Verification items for the finished model (mm, model axes). Face numbers are marked on the shaded views. A direction names the side the tool comes from. Coordinates: 2 decimals unless noted, no trailing zeros. Order: outer loops, then holes, each group sorted by start corner. A loop starts at its lowest first (then second) coordinate and runs counter-clockwise, first axis right, second up.
Q1. Draft check along Z on the marked faces 4, 5, 6 and 7. Enter one of: pulls with the +Z half, pulls with the -Z half, needs draft (parallel to the pull), parting line crosses it, or undercut.
Q2. Depth check by flat-ended pin: P1, Ø0.8, axis at x = 8, z = 20, coming from the -Y side; P2, Ø0.7, axis at x = -0.5, z = 12, coming from the +Y side; P3, Ø2.5, axis at y = 73.19, z = 6.34, coming from the -X side; P4, Ø3.5, axis at x = 0, z = 12, coming from the +Y side. Enter the tip coordinate at first touch or a pass-through.
Q3. Thickness scan on line 1 (X direction, y = 2, z = 20); line 2 (Z direction, x = 0, y = 7.75); line 3 (X direction, y = 34.5, z = 23). Record the ranges inside material, lowest first.
Q4. Cross-section at D-D, the plane z = 35. Record the boundary of the cut face in (x, y), and give its area (3 significant figures).
Q5. Cross-section at A-A, the plane x = -3. Record the boundary of the cut face in (y, z), and give its area (3 significant figures).
Q6. Cross-section at B-B, the plane x = 24. Count the separate pieces of the cut face and the enclosed holes in it, and give its area (3 significant figures).
Q7. Set-up check for the marked faces 1, 2 and 3: record each of +Z, -Z, +X, -X, +Y, -Y from which the full face is reachable in a straight line by a thin tool's end or side.
from build123d import *

# Parameters (mm, degrees)
DODANIE_WYCI_GNI_CIE1_DEPTH = 40
SZKIC2_R                    = 4.25
WYTNIJ_WYCI_GNI_CIE1_DEPTH  = 59
SZKIC3_R                    = 4.25
SZKIC3_R_2                  = 0.65
WYTNIJ_WYCI_GNI_CIE2_DEPTH  = 11
SZKIC4_R                    = 0.75
WYTNIJ_WYCI_GNI_CIE3_DEPTH  = 59
SZKIC3_3_R                  = 1.15
WYTNIJ_WYCI_GNI_CIE4_DEPTH  = 4


with BuildPart() as part:
    # Szkic1 → Dodanie-wyci_gni_cie1 (new body)
    with BuildSketch(Plane.XY):
        Polygon((21, 10), (-21, 10), (-21, 80), (-29, 80), (-29, 0), (29, 0), (29, 80), (21, 80), align=None)
    extrude(amount=DODANIE_WYCI_GNI_CIE1_DEPTH)

    # Szkic2 → Wytnij-wyci_gni_cie1 (cut, through all)
    with BuildSketch(Plane(origin=(29, 0, 0), x_dir=(0, 0, -1), z_dir=(1, 0, 0))):
        with BuildLine():
            ThreePointArc((-23.582337322, 70.675180947), (-10.416972499, 79.431921725), (0, 67.536795667))
            Line((0, 67.536795667), (0, 80))
            Line((0, 80), (-40, 80))
            Line((-40, 80), (-40, 14.688889066))
            ThreePointArc((-40, 14.688889066), (-38.089938994, 25.648227934), (-32.584991767, 35.315233546))
            ThreePointArc((-32.584991767, 35.315233546), (-26.211441646, 46.507556061), (-24, 59.196123761))
            Line((-24, 59.196123761), (-24, 67.536795667))
            ThreePointArc((-24, 67.536795667), (-23.895126058, 69.119823168), (-23.582337322, 70.675180947))
        make_face()
        with Locations((-12, 67.536795667)):
            Circle(SZKIC2_R)
    extrude(amount=-WYTNIJ_WYCI_GNI_CIE1_DEPTH, mode=Mode.SUBTRACT)

    # Szkic3 → Wytnij-wyci_gni_cie2 (cut, through all)
    with BuildSketch(Plane(origin=(0, 10, 0), x_dir=(1, 0, 0), z_dir=(0, 1, 0))):
        with Locations((0, -20)):
            Circle(SZKIC3_R)
        with Locations((5.656854249, -25.656854249)):
            Circle(SZKIC3_R_2)
        with Locations((8, -20)):
            Circle(SZKIC3_R_2)
        with Locations((0, -28)):
            Circle(SZKIC3_R_2)
        with Locations((-5.656854249, -25.656854249)):
            Circle(SZKIC3_R_2)
        with Locations((-8, -20)):
            Circle(SZKIC3_R_2)
        with Locations((-5.656854249, -14.343145751)):
            Circle(SZKIC3_R_2)
        with Locations((0, -12)):
            Circle(SZKIC3_R_2)
        with Locations((5.656854249, -14.343145751)):
            Circle(SZKIC3_R_2)
    extrude(amount=-WYTNIJ_WYCI_GNI_CIE2_DEPTH, mode=Mode.SUBTRACT)

    # Szkic4 → Wytnij-wyci_gni_cie3 (cut, through all)
    with BuildSketch(Plane.ZY.offset(29)):
        with Locations((12, 59.536795667)):
            Circle(SZKIC4_R)
        with Locations((6.343145751, 61.879941418)):
            Circle(SZKIC4_R)
        with Locations((4, 67.536795667)):
            Circle(SZKIC4_R)
        with Locations((6.343145751, 73.193649917)):
            Circle(SZKIC4_R)
        with Locations((12, 75.536795667)):
            Circle(SZKIC4_R)
        with Locations((17.656854249, 73.193649917)):
            Circle(SZKIC4_R)
        with Locations((20, 67.536795667)):
            Circle(SZKIC4_R)
        with Locations((17.656854249, 61.879941418)):
            Circle(SZKIC4_R)
    extrude(amount=-WYTNIJ_WYCI_GNI_CIE3_DEPTH, mode=Mode.SUBTRACT)

    # Szkic3_3 → Wytnij-wyci_gni_cie4 (cut)
    with BuildSketch(Plane(origin=(0, 10, 0), x_dir=(1, 0, 0), z_dir=(0, 1, 0))):
        with Locations((8, -20)):
            Circle(SZKIC3_3_R)
        with Locations((5.656854249, -25.656854249)):
            Circle(SZKIC3_3_R)
        with Locations((0, -28)):
            Circle(SZKIC3_3_R)
        with Locations((-5.656854249, -25.656854249)):
            Circle(SZKIC3_3_R)
        with Locations((-8, -20)):
            Circle(SZKIC3_3_R)
        with Locations((-5.656854249, -14.343145751)):
            Circle(SZKIC3_3_R)
        with Locations((0, -12)):
            Circle(SZKIC3_3_R)
        with Locations((5.656854249, -14.343145751)):
            Circle(SZKIC3_3_R)
    extrude(amount=-WYTNIJ_WYCI_GNI_CIE4_DEPTH, mode=Mode.SUBTRACT)


solid = part.part
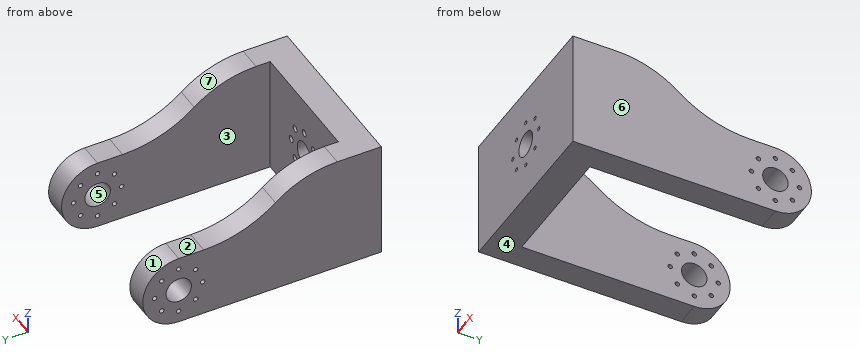
Check values:
1. face 4: pulls with the -Z half
1. face 5: undercut
1. face 6: needs draft
1. face 7: pulls with the +Z half
2. P1: passes through
2. P2: stops at y = 6
2. P3: stops at x = -29
2. P4: stops at y = 10
3. line 1: x = -29 to -8.65, -7.35 to -4.25, 4.25 to 7.35, 8.65 to 29
3. line 2: z = 0 to 10.85, 13.15 to 15.75, 24.25 to 26.85, 29.15 to 40
3. line 3: x = -29 to -21, 21 to 29
4. outline: (-29, 0) - (29, 0) - (29, 31.98) - (21, 31.98) - (21, 10) - (-21, 10) - (-21, 31.98) - (-29, 31.98) - close
4. area: 932 mm2
5. outline: (0, 0) - (10, 0) - (10, 16.99) - (0, 16.99) - close; (0, 23.01) - (10, 23.01) - (10, 40) - (0, 40) - close
5. area: 340 mm2
6. separate pieces: 1
6. enclosed holes: 9
6. area: 2,360 mm2
7. face 1: +X, -X, +Y
7. face 2: +Z, +X, -X, +Y
7. face 3: +Z, -Z, +Y
